Can you work these out from the drawing? Everything is in mm from the part's minimum corner. Round coordinates to 2 decimals unless told otherwise and drop trailing zeros. Loops run counter-clockwise (first coordinate to the right, second up) from the corner with the lowest first, then second, coordinate; pieces in that order, holes last. Notation, with made-up numbers: (8.25, 20.25) -> (60.25, 20.25) arc R19 ccw to (60.25, 55.25) -> close; hole circle Ø10 at (9.5, 52.25). An arc over 180 degrees is marked (long way). Answer as a JSON object with one key per item and string values.
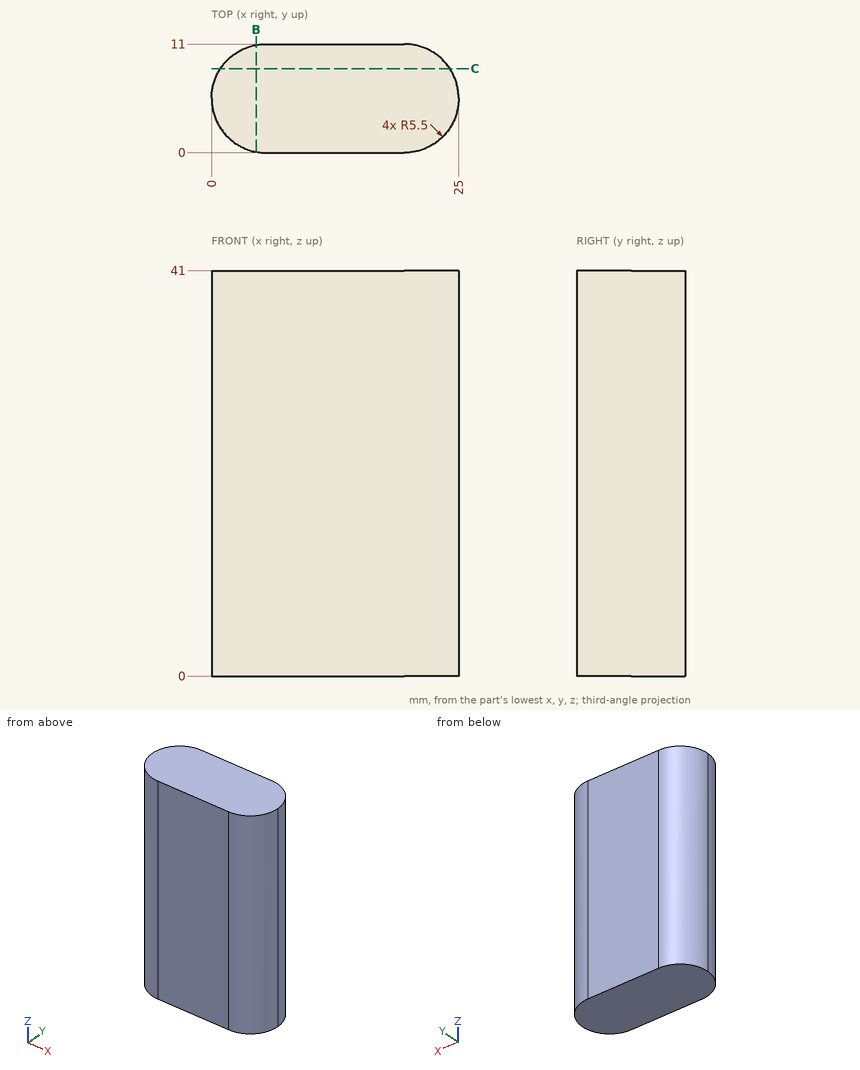
Q1. I'm going to push a flat-ended pin straight in: pin 1 (2 mm diameter, centred on x = 21.5, z = 10, fed in from +Y). Where does the tip first touch, or does it pass through?
Determined:
{"pin 1": "y = 10.91"}
Q2. I want a section at C-C, the plane y = 8.5. Write out the boundary of the cut face in (x, z), then the cut area to 3 significant figures.
Determined:
{"outline": "(0.89, 0) -> (24.11, 0) -> (24.11, 41) -> (0.89, 41) -> close", "area": "952 mm²"}
Q3. If I drill on L1, parallel to X at y = 5, z = 15; L2, parallel to X at y = 8.75, z = 27.5; L3, parallel to Y at x = 1, z = 27.5, over which ranges is the centre line in solid material (lowest first)? Write a range as [from, to].
Determined:
{"L1": "[0.02, 24.98]", "L2": "[1.06, 23.94]", "L3": "[2.34, 8.66]"}
Q4. I want a section at B-B, the plane x = 4.5. Write out the boundary of the cut face in (y, z).
Determined:
{"outline": "(0.09, 0) -> (10.91, 0) -> (10.91, 41) -> (0.09, 41) -> close"}
